The model under review builds one solid part; all positions refer to its coordinate system, in mm. A direction names the side the tool comes from. Round coordinates to 2 decimals unless told otherwise and drop trailing zeros. Order: outer loops, then holes, each group sorted by start corner. A loop starts at its lowest first (then second) coordinate and runs counter-clockwise, first axis right, second up. Notation, with made-up numbers: M -19.5,45.25 L 20.5,45.25 A13 ccw 20.5,58.25 Z; hole C -4.5,-18 d7. An arc over 180 degrees is marked long. Answer as a JSON object with one key per item and string values. Group by question number.
1) Consider section D-D, the plane x = -38.5. Write out the cut boundary in (y, z).
2) To check wall thickness, follow line 1 (X direction, y = -11.5, z = -17); line 2 (X direction, y = -2, z = 34.5); line 3 (Z direction, x = 94.5, y = -1.75). State the ranges of each line that lie inside material, in increasing order.
3) Consider section C-C, the plane y = -22. Write out the cut boundary in (x, z), then the cut area to 3 significant figures.
4) Consider section B-B, the plane z = 40. Write out the cut boundary in (x, y), then the cut area to 3 significant figures.
5) The part is to be moulded in two halves that separate along Z. For faces 4 (the flat face through (-74.727, -13, 9)), 5 (the flat face through (-2, -13, -42.189)), 6 (the flat face through (-110, -13, 46.711)), 7 (the flat face through (18.796, -16, 12)), say which applies: +Z half, -Z half, draft (parallel to the pull), parting line (faces both ways), or undercut.
6) Consider section A-A, the plane x = 126.5. Write out the cut boundary in (y, z).
7) For faces 1 (the flat face through (-25, -6.35, 12)), 2 (the flat face through (32, -25.4, 9)), 3 (the flat face through (15.926, -3, -9)), list the 3-axis set-ups (+Z, -Z, +X, -X, +Y, -Y) from which the entire face can be reached by the end or side of a thin tool; tool diameter is ignored.
8) Insertion check: pin 1 Ø10 at (x, y) = (-17, -18) entering from +Z. The pin has a flat end and moves straight along its axis. Give the tip position at first contact, or say it passes through.
```python
from build123d import *

# Parameters (mm, degrees)
F0_W     = 7.8232
F0_H     = 6.35
F0_W_2   = 69.85
F0_W_3   = 55.9308
F0_H_2   = 76.2
F0_W_4   = 7.7978
F0_H_3   = 12.7
F0_W_5   = 85.725
F1_DEPTH = 25.4
F0_W_6   = 16.764
F0_H_4   = 0.762
F0_H_5   = 13.4315382606
F0_W_7   = 66.0908
F0_W_8   = 2.8702
F0_H_6   = 4.9097025247
F0_H_7   = 5.1918955931
F2_DEPTH = 6.35


with BuildPart() as f1:
    # F0 (on Front) → F1 (new body)
    with BuildSketch(Plane.XZ):
        with Locations((148.4884, 56.2362195122)):
            Rectangle(F0_W, F0_H)
        with Locations((109.6518, 56.2362195122)):
            Rectangle(F0_W_2, F0_H)
        with Locations((148.4884, 49.8862195122)):
            Rectangle(F0_W, F0_H)
        with Locations((46.7614, 56.2362195122)):
            Rectangle(F0_W_3, F0_H)
        with Locations((109.6518, 49.8862195122)):
            Rectangle(F0_W_2, F0_H)
        with Locations((148.4884, 8.6112195122)):
            Rectangle(F0_W, F0_H_2)
        with Locations((46.7614, 49.8862195122)):
            Rectangle(F0_W_3, F0_H)
        with Locations((148.4884, -32.6637804878)):
            Rectangle(F0_W, F0_H)
        with Locations((-70.8279, 56.2362195122)):
            Rectangle(F0_W_4, F0_H)
        Polygon((74.7268, -2.1837804878), (74.7268, 46.7112195122), (18.796, 46.7112195122), (18.796, 3.0081151053), (18.796, -2.1837804878), align=None)
        with Locations((109.6518, -32.6637804878)):
            Rectangle(F0_W_2, F0_H)
        with Locations((148.4884, -39.0137804878)):
            Rectangle(F0_W, F0_H)
        with Locations((-109.6518, 56.2362195122)):
            Rectangle(F0_W_2, F0_H)
        with Locations((-70.8279, 49.8862195122)):
            Rectangle(F0_W_4, F0_H)
        with Locations((46.7614, -8.5337804878)):
            Rectangle(F0_W_3, F0_H_3)
        with Locations((109.6518, -39.0137804878)):
            Rectangle(F0_W_2, F0_H)
        Polygon((18.796, -29.4887804878), (74.7268, -29.4887804878), (74.7268, -14.8837804878), (18.796, -14.8837804878), (18.796, -28.3153187484), align=None)
        with Locations((46.7614, -32.6637804878)):
            Rectangle(F0_W_3, F0_H)
        with Locations((-148.4884, 56.2362195122)):
            Rectangle(F0_W, F0_H)
        with Locations((-109.6518, 49.8862195122)):
            Rectangle(F0_W_2, F0_H)
        Polygon((-66.929, 2.7259220369), (-66.929, 46.7112195122), (-74.7268, 46.7112195122), (-74.7268, -2.1837804878), (-66.929, -2.1837804878), align=None)
        with Locations((46.7614, -39.0137804878)):
            Rectangle(F0_W_3, F0_H)
        with Locations((-148.4884, 49.8862195122)):
            Rectangle(F0_W, F0_H)
        with Locations((-24.0665, -39.0137804878)):
            Rectangle(F0_W_5, F0_H)
        Polygon((-74.7268, -29.4887804878), (-66.929, -29.4887804878), (-66.929, -28.3153187484), (-66.929, -14.8837804878), (-74.7268, -14.8837804878), align=None)
        with Locations((-70.8279, -32.6637804878)):
            Rectangle(F0_W_4, F0_H)
        with Locations((-148.4884, 8.6112195122)):
            Rectangle(F0_W, F0_H_2)
        with Locations((-70.8279, -8.5337804878)):
            Rectangle(F0_W_4, F0_H_3)
        with Locations((-70.8279, -39.0137804878)):
            Rectangle(F0_W_4, F0_H)
        with Locations((-109.6518, -32.6637804878)):
            Rectangle(F0_W_2, F0_H)
        with Locations((-148.4884, -32.6637804878)):
            Rectangle(F0_W, F0_H)
        with Locations((-109.6518, -39.0137804878)):
            Rectangle(F0_W_2, F0_H)
        with Locations((-148.4884, -39.0137804878)):
            Rectangle(F0_W, F0_H)
    extrude(amount=F1_DEPTH)

    # F0 (on Front) → F2 (join)
    with BuildSketch(Plane.XZ):
        with Locations((7.5438, -2.5647804878)):
            Rectangle(F0_W_6, F0_H_4)
        with Locations((7.5438, -21.5995496181)):
            Rectangle(F0_W_6, F0_H_5)
        Polygon((-66.929, -29.4887804878), (18.796, -29.4887804878), (18.796, -28.3153187484), (15.9258, -28.3153187484), (-0.8382, -28.3153187484), (-66.929, -28.3153187484), align=None)
        with Locations((-24.0665, -32.6637804878)):
            Rectangle(F0_W_5, F0_H)
        with Locations((-33.8836, -21.5995496181)):
            Rectangle(F0_W_7, F0_H_5)
        with Locations((17.3609, -21.5995496181)):
            Rectangle(F0_W_8, F0_H_5)
        Polygon((18.796, -14.8837804878), (18.796, -2.1837804878), (15.9258, -2.1837804878), (15.9258, -2.9457804878), (15.9258, -14.8837804878), align=None)
        Polygon((-0.8382, -2.1837804878), (-66.929, -2.1837804878), (-66.929, -14.8837804878), (-0.8382, -14.8837804878), (-0.8382, -2.9457804878), align=None)
        with Locations((-33.8836, 0.2710707746)):
            Rectangle(F0_W_7, F0_H_6)
        Polygon((15.9258, -2.1837804878), (15.9258, 3.0081151053), (-0.8382, 3.0081151053), (-0.8382, 2.7259220369), (-0.8382, -2.1837804878), align=None)
        with Locations((17.3609, 0.4121673088)):
            Rectangle(F0_W_8, F0_H_7)
        Polygon((18.796, 3.0081151053), (18.796, 46.7112195122), (-66.929, 46.7112195122), (-66.929, 2.7259220369), (-0.8382, 2.7259220369), (-0.8382, 3.0081151053), (15.9258, 3.0081151053), align=None)
        with Locations((-24.0665, 49.8862195122)):
            Rectangle(F0_W_5, F0_H)
        with Locations((-24.0665, 56.2362195122)):
            Rectangle(F0_W_5, F0_H)
    extrude(amount=F2_DEPTH)


solid = f1.part
```
Results list:
{
 "1": {"outline": "M -25.4,-42.19 L 0,-42.19 L 0,59.41 L -6.35,59.41 L -6.35,-35.84 L -25.4,-35.84 Z"},
 "2": {"line 1": "-152.4 to -144.58, -74.73 to -66.93, 18.8 to 74.73, 144.58 to 152.4", "line 2": "-152.4 to -144.58, -74.73 to 74.73, 144.58 to 152.4", "line 3": "-42.19 to -29.49, 46.71 to 59.41"},
 "3": {"outline": "M -152.4,-42.19 L 152.4,-42.19 L 152.4,59.41 L 18.8,59.41 L 18.8,-35.84 L -66.93,-35.84 L -66.93,59.41 L -152.4,59.41 Z; hole M -144.58,-29.49 L -74.73,-29.49 L -74.73,46.71 L -144.58,46.71 Z; hole M 74.73,-29.49 L 144.58,-29.49 L 144.58,46.71 L 74.73,46.71 Z", "area": "12,200 mm^2"},
 "4": {"outline": "M -152.4,-25.4 L -144.58,-25.4 L -144.58,0 L -152.4,0 Z; M -74.73,-25.4 L -66.93,-25.4 L -66.93,-6.35 L 18.8,-6.35 L 18.8,-25.4 L 74.73,-25.4 L 74.73,0 L -74.73,0 Z; M 144.58,-25.4 L 152.4,-25.4 L 152.4,0 L 144.58,0 Z", "area": "2,560 mm^2"},
 "5": {"face 4": "undercut", "face 5": "-Z half", "face 6": "undercut", "face 7": "draft"},
 "6": {"outline": "M -25.4,-42.19 L 0,-42.19 L 0,-29.49 L -25.4,-29.49 Z; M -25.4,46.71 L 0,46.71 L 0,59.41 L -25.4,59.41 Z"},
 "7": {"face 1": "+Z, -Y", "face 2": "+Z, -Z, +X, -X, -Y", "face 3": "+Y, -Y"},
 "8": {"pin 1": "z = -35.84"}
}
